Verification items for the finished model (mm, model axes). Coordinates: 2 decimals unless noted, no trailing zeros. Loops run counter-clockwise (first coordinate to the right, second up) from the corner with the lowest first, then second, coordinate; pieces in that order, holes last.
Q1. Sectioned sample at B-B (x = -50.5). Enter the section's corners in (y, z).
Q2. Material ranges on probe 1 along X at (y, z) = (-32.5, 2.1); probe 2 along Y at (x, z) = (-11, 2.85); probe 3 along Y at (x, z) = (-81.5, 1.05), recorded low to high.
Q3. Go/stop test with flat-tipped pins: P1, Ø3, axis at y = 43, z = 4, coming from the +X side; P2, Ø2, axis at x = -55.5, z = 2, coming from the -Y side. Record where each tip stops, or that it passes through.
Q4. Sectioned sample at C-C (y = 58). Enter the section's corners in (x, z), then the cut area to 3 significant figures.
Q5. Sectioned sample at A-A (z = 4.15). Enter the section's corners in (x, y).
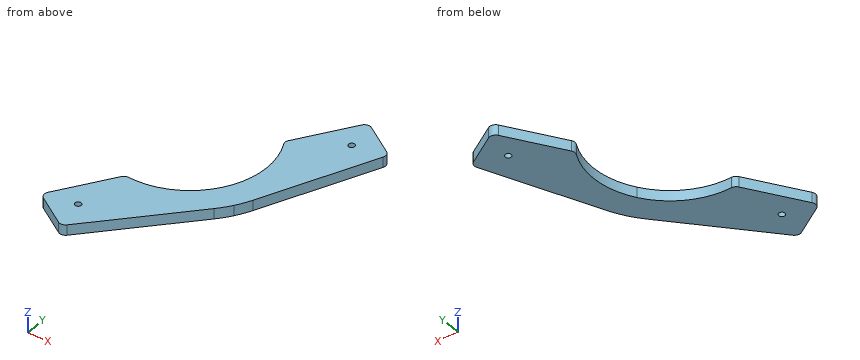
```python
from build123d import *

# Parameters (mm, degrees)
SKETCH1_R           = 1.5
BOSS_EXTRUDE1_DEPTH = 5


with BuildPart() as part:
    # Sketch1 → Boss-Extrude1 (new body)
    # profile 1 of 2: a face of its own
    with BuildSketch(Plane.XY):
        with BuildLine():
            ThreePointArc((-72.013621978, -46.836846361), (-70.000170189, -47.302108237), (-68.163524501, -46.354907448))
            Line((-68.163524501, -46.354907448), (-28.639229463, -3.331157144))
            ThreePointArc((-28.639229463, -3.331157144), (-25.987391066, -0.195217043), (-23.601858593, 3.14777593))
            Line((-23.601858593, 3.14777593), (-34.401340039, 10.203355318))
            ThreePointArc((-34.401340039, 10.203355318), (-48.850216004, -2.67902279), (-67.821167684, -6.529824621))
            ThreePointArc((-67.821167684, -6.529824621), (-69.355206904, -6.841210213), (-70.523579623, -7.882911947))
            Line((-70.523579623, -7.882911947), (-87.164902157, -33.35461938))
            ThreePointArc((-87.164902157, -33.35461938), (-87.589542424, -35.611111919), (-86.29422726, -37.506959108))
            Line((-86.29422726, -37.506959108), (-72.013621978, -46.836846361))
        make_face()
        with Locations((-73.020492871, -32.63009114)):
            Circle(SKETCH1_R, mode=Mode.SUBTRACT)
    # profile 2 of 2: a face of its own
    with BuildSketch(Plane.XY):
        with BuildLine():
            Line((-34.401340039, 10.203355318), (-23.601858593, 3.14777593))
            ThreePointArc((-23.601858593, 3.14777593), (-21.49872615, 6.675268117), (-19.692182619, 10.363461126))
            Line((-19.692182619, 10.363461126), (3.830578313, 63.841425809))
            ThreePointArc((3.830578313, 63.841425809), (3.960207556, 65.903864408), (2.725322858, 67.560824426))
            Line((2.725322858, 67.560824426), (-11.555282424, 76.890711678))
            ThreePointArc((-11.555282424, 76.890711678), (-13.811774964, 77.315351945), (-15.707622153, 76.020036781))
            Line((-15.707622153, 76.020036781), (-32.348944687, 50.548329348))
            ThreePointArc((-32.348944687, 50.548329348), (-32.833563081, 49.059913302), (-32.502490474, 47.530002114))
            ThreePointArc((-32.502490474, 47.530002114), (-28.408225903, 28.610100423), (-34.401340039, 10.203355318))
        make_face()
        with Locations((-10.689254116, 62.775972546)):
            Circle(SKETCH1_R, mode=Mode.SUBTRACT)
    extrude(amount=BOSS_EXTRUDE1_DEPTH)


solid = part.part
```
Geometry check:
1. outline: (-27.13, 0) - (-3.45, 0) - (-3.45, 5) - (-27.13, 5) - close
2. probe 1: x = -86.61 to -74.51, -71.53 to -55.44
2. probe 2: y = 30.12 to 61.31, 64.24 to 76.53
2. probe 3: y = -40.64 to -24.68
3. P1: stops at x = -4.68
3. P2: stops at y = -33.66
4. outline: (-27.48, 0) - (1.26, 0) - (1.26, 5) - (-27.48, 5) - close
4. area: 144 mm2
5. outline: (-87.16, -33.35) arc R3 ccw to (-86.29, -37.51) - (-72.01, -46.84) arc R3 ccw to (-68.16, -46.35) - (-28.64, -3.33) arc R50 ccw to (-19.69, 10.36) - (3.83, 63.84) arc R3 ccw to (2.73, 67.56) - (-11.56, 76.89) arc R3 ccw to (-15.71, 76.02) - (-32.35, 50.55) arc R3 ccw to (-32.5, 47.53) arc R37.1 cw to (-67.82, -6.53) arc R3 ccw to (-70.52, -7.88) - close; hole circle Ø3 at (-73.02, -32.63); hole circle Ø3 at (-10.69, 62.78)
